Read the model definition and answer for the solid it produces. Units are mm, in the model's axes. A direction names the side the tool comes from. Coordinates: 2 decimals unless noted, no trailing zeros. Order: outer loops, then holes, each group sorted by start corner. A loop starts at its lowest first (then second) coordinate and runs counter-clockwise, first axis right, second up.
from build123d import *

# Parameters (mm, degrees)
SKETCH2_W               = 100
SKETCH2_H               = 10
BOSS_EXTRUDE2_DEPTH     = 12.5
CUT_EXTRUDE3_DEPTH      = 53.5
CUT_EXTRUDE3_DEPTH_BACK = 53.5
SKETCH6_W               = 60
SKETCH6_H               = 7.5
FILLET2_R               = 3


with BuildPart() as part:
    # Sketch2 → Boss-Extrude2 (new, symmetric)
    with BuildSketch(Plane(origin=(0, 0, 0), x_dir=(1, 0, 0), z_dir=(0, 1, 0))):
        Rectangle(SKETCH2_W, SKETCH2_H)
    extrude(amount=BOSS_EXTRUDE2_DEPTH, both=True)

    # Sketch6 → Cut-Extrude3 (cut, two sides: drawn at the far end of the back side and taken through both)
    with BuildSketch(Plane.XY.offset(5).offset(-CUT_EXTRUDE3_DEPTH_BACK)):
        with Locations((-20, 8.75)):
            Rectangle(SKETCH6_W, SKETCH6_H)
        with Locations((-20, -8.75)):
            Rectangle(SKETCH6_W, SKETCH6_H)
    extrude(amount=CUT_EXTRUDE3_DEPTH + CUT_EXTRUDE3_DEPTH_BACK, mode=Mode.SUBTRACT)

    # Fillet2
    fillet2_edges = [part.edges().sort_by_distance(p)[0] for p in [
        (10, 5, 0),
        (10, 12.5, 0),
        (10, -12.5, 0),
        (10, -5, 0),
    ]]
    fillet(fillet2_edges, radius=FILLET2_R)


solid = part.part
Q1. Which of the six approach directions +Z, -Z, +X, -X, +Y, -Y give full straight-line access (tool end or side, diameter ignored) to faces 1 (the flat face through (-22, 5, 0)), 2 (the flat face through (-22, -5, 0)), 3 (the flat face through (10, 0, 5))?
Q2. The part is cut by section B-B, the plane x = -11.5. Determine the outline of the cut face in (y, z), then the cut area to 3 significant figures.
Q3. The part is cut by section C-C, the plane y = -10.5. Determine the outline of the cut face in (x, z), then the cut area to 3 significant figures.
Q4. The part is cut by section A-A, the plane z = -2.5. Determine the outline of the cut face in (x, y), then the cut area to 3 significant figures.
Q5. Each of these flat-tipped pins is pushed along its axis until it touches: P1, Ø1.6, axis at y = 9, z = 0.5, coming from the -X side; P2, Ø10, axis at x = -35, y = -6, coming from the +Z side; P3, Ø3, axis at x = -9, z = -2.5, coming from the -Y side; P4, Ø5, axis at x = -20, z = -1.5, coming from the +Y side. Where does it stop, or does it pass through?
Q6. Straight lines are drawn through the part: L1, parallel to Y at x = -37, z = -1.5; L2, parallel to X at y = -8.5, z = 4.75; L3, parallel to X at y = -6.5, z = -4. For each, find the intervals that lie inside material, in ascending order.
Computed values:
1. face 1: +Z, -Z, -X, +Y
1. face 2: +Z, -Z, -X, -Y
1. face 3: +Z, +X, -X, +Y, -Y
2. outline: (-5, -5) - (5, -5) - (5, 5) - (-5, 5) - close
2. area: 100 mm2
3. outline: (10.17, -5) - (50, -5) - (50, 5) - (10.17, 5) - close
3. area: 398 mm2
4. outline: (-50, -5) - (7, -5) arc R3 cw to (10, -8) - (10, -9.5) arc R3 ccw to (13, -12.5) - (50, -12.5) - (50, 12.5) - (13, 12.5) arc R3 ccw to (10, 9.5) - (10, 8) arc R3 cw to (7, 5) - (-50, 5) - close
4. area: 1,600 mm2
5. P1: stops at x = 10
5. P2: stops at z = 5
5. P3: stops at y = -5
5. P4: stops at y = 5
6. L1: y = -5 to 5
6. L2: x = 10 to 50
6. L3: x = 9.6 to 50
